Can you work these out from the model? Positions are in its coordinate system, mm. Face numbers are marked on the shaded views. A direction names the side the tool comes from. Coordinates: 2 decimals unless noted, no trailing zeros. Order: outer loops, then holes, each group sorted by start corner. A loop starts at its lowest first (then second) coordinate and runs counter-clockwise, first axis right, second up. Notation, with made-up numbers: (-26, 63.5) -> (-1, 63.5) arc R10 ccw to (-1, 76.5) -> close; hole circle Ø2 at (42.5, -21.75). An arc over 180 degrees is marked (long way). Return JSON: item names as keys, results as strings. Group by question number.
1) If we section it at A-A, the plane z = -28.5: Please give me the cut outline in (x, y), then the cut area to 3 significant figures.
2) For the marked faces 5 and 6, which set-ups out of +Z, -Z, +X, -X, +Y, -Y let a thin tool reach every point of the face, with its end or its side?
3) If I drill on probe 1 along Z at (x, y) = (7.5, 1.6); probe 2 along Z at (x, y) = (11.5, 3.5); probe 3 along X at (y, z) = (3.4, -27.5), over which ranges is the centre line in solid material (lowest first)? Write a range as from..to.
4) If we section it at C-C, the plane y = 2.35: Please give me the cut outline in (x, z).
5) If we section it at B-B, the plane x = 5.75: Please give me the cut outline in (y, z), then the cut area to 3 significant figures.
6) Thinking about a two-plate mould opening in X: for the marked faces 1, 2, 3 and 4, which applies, +X half, -X half, draft (parallel to the pull), parting line (faces both ways), or undercut?
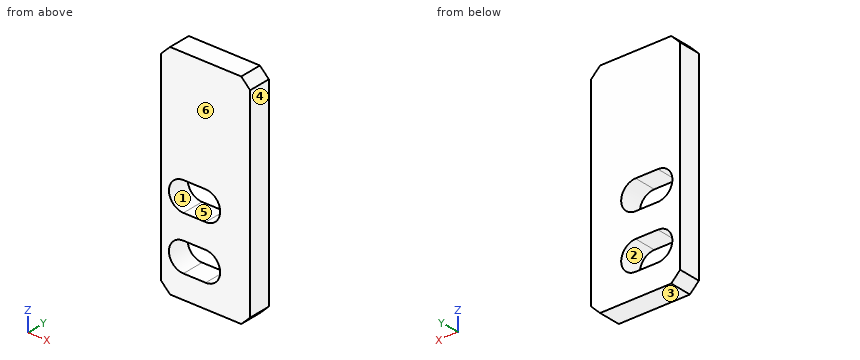
from build123d import *

# Parameters (mm, degrees)
BOSS_EXTRUDE1_DEPTH = 5
SKETCH1_5_OUTSIDE_W = 32.632
SKETCH1_5_OUTSIDE_H = 61.632
CUT_EXTRUDE5_DEPTH  = 5


with BuildPart() as part:
    # Sketch1 → Boss-Extrude1 (new body)
    with BuildSketch(Plane(origin=(0, 0, 0), x_dir=(1, 0, 0), z_dir=(0, 1, 0))):
        Polygon((0, 47), (2, 49), (18, 49), (20, 47), (20, 2), (18, 0), (2, 0), (0, 2), align=None)
    extrude(amount=BOSS_EXTRUDE1_DEPTH)

    # Sketch1<5> outside → Cut-Extrude5 (cut)
    # profile 1 of 3: a face of its own
    with BuildSketch(Plane(origin=(0, 0, 0), x_dir=(1, 0, 0), z_dir=(0, 1, 0))):
        with Locations((10, 24.5)):
            Rectangle(SKETCH1_5_OUTSIDE_W, SKETCH1_5_OUTSIDE_H)
        Polygon((0, 47), (2, 49), (18, 49), (20, 47), (20, 2), (18, 0), (2, 0), (0, 2), align=None, mode=Mode.SUBTRACT)
    # profile 2 of 3: a face of its own
    with BuildSketch(Plane(origin=(0, 0, 0), x_dir=(1, 0, 0), z_dir=(0, 1, 0))):
        with BuildLine():
            Line((10, 37.25), (5, 37.25))
            ThreePointArc((5, 37.25), (1.75, 40.5), (5, 43.75))
            Line((5, 43.75), (10, 43.75))
            ThreePointArc((10, 43.75), (13.25, 40.5), (10, 37.25))
        make_face()
    # profile 3 of 3: a face of its own
    with BuildSketch(Plane(origin=(0, 0, 0), x_dir=(1, 0, 0), z_dir=(0, 1, 0))):
        with BuildLine():
            Line((5, 31.75), (10, 31.75))
            ThreePointArc((10, 31.75), (13.25, 28.5), (10, 25.25))
            Line((10, 25.25), (5, 25.25))
            ThreePointArc((5, 25.25), (1.75, 28.5), (5, 31.75))
        make_face()
    extrude(amount=CUT_EXTRUDE5_DEPTH, mode=Mode.SUBTRACT)


solid = part.part
Result sheet:
{
 "1": {"outline": "(0, 0) -> (1.75, 0) -> (1.75, 5) -> (0, 5) -> close; (13.25, 0) -> (20, 0) -> (20, 5) -> (13.25, 5) -> close", "area": "42.5 mm2"},
 "2": {"face 5": "+Y, -Y", "face 6": "+Z, -Z, +X, -X, -Y"},
 "3": {"probe 1": "z = -49..-43.75, -37.25..-31.75, -25.25..0", "probe 2": "z = -49..-43.38, -37.62..-31.38, -25.62..0", "probe 3": "x = 0..1.91, 13.09..20"},
 "4": {"outline": "(0, -47) -> (2, -49) -> (18, -49) -> (20, -47) -> (20, -2) -> (18, 0) -> (2, 0) -> (0, -2) -> close; hole (5, -43.75) -> (10, -43.75) arc R3.25 ccw to (10, -37.25) -> (5, -37.25) arc R3.25 ccw to start; hole (5, -31.75) -> (10, -31.75) arc R3.25 ccw to (10, -25.25) -> (5, -25.25) arc R3.25 ccw to start"},
 "5": {"outline": "(0, -49) -> (5, -49) -> (5, -43.75) -> (0, -43.75) -> close; (0, -37.25) -> (5, -37.25) -> (5, -31.75) -> (0, -31.75) -> close; (0, -25.25) -> (5, -25.25) -> (5, 0) -> (0, 0) -> close", "area": "180 mm2"},
 "6": {"face 1": "undercut", "face 2": "undercut", "face 3": "draft", "face 4": "+X half"}
}
